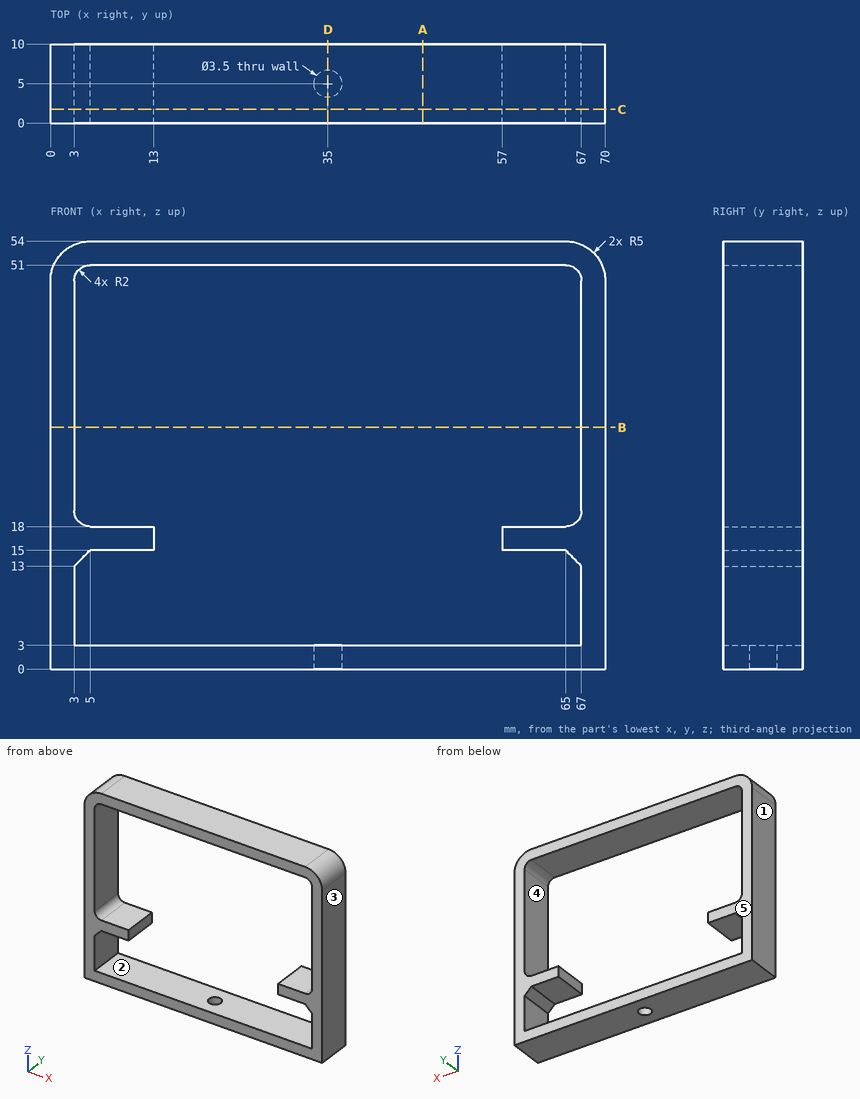
Study the drawing (mm; zero at the part's minimum x, y, z) and answer. A direction names the side the tool comes from. Round coordinates to 2 decimals unless told otherwise and drop trailing zeros. Write each loop counter-clockwise with the first axis right and the second up, starting at its lowest first coordinate (ties: lowest second). Pieces come first, ordered by that corner, then holes. Notation, with made-up numbers: (53.5, -23.75) -> (98.5, -23.75) arc R17 cw to (98.5, 5.25) -> close; hole circle Ø10 at (-4.75, -5). An arc over 180 degrees is marked (long way). Write item = value, one per line.
1) Which of the six approach directions +Z, -Z, +X, -X, +Y, -Y give full straight-line access (tool end or side, diameter ignored) to the marked faces 4 and 5?
Check values:
face_4 = +Y, -Y
face_5 = +Z, -Z, +X, -X, +Y
2) For a pull along X with two mould halves and no side action, classify the marked faces 1, 2 and 3 as released by +X, released by -X, zero draft, split by the parting line, or undercut.
Check values:
face_1 = released by -X
face_2 = undercut
face_3 = released by +X
3) Given pin 1 (2.5 mm diameter, centred on x = 61, y = 6, fed in from -Z); pin 2 (8 mm diameter, centred on x = 8.5, z = 32, fed in from +Y), each flat-ended and moving along its own axis, determine where each tip first touches the part or whether it passes through.
Check values:
pin_1 = 0
pin_2 = through
4) Section B-B on z = 30.5 is taken. Write down the section's boundary in (x, y).
Check values:
outline = (0, 0) -> (3, 0) -> (3, 10) -> (0, 10) -> close; (67, 0) -> (70, 0) -> (70, 10) -> (67, 10) -> close
5) Straight lines are drawn through the part: line 1 along Z through (x, y) = (60, 5); line 2 along Z through (x, y) = (48, 8); line 3 along Y through (x, z) = (35, 1.1). For each, find the intervals that lie inside material, in ascending order. Write a range as [from, to].
Check values:
line_1 = [0, 3], [15, 18], [51, 54]
line_2 = [0, 3], [51, 54]
line_3 = [0, 3.25], [6.75, 10]
6) Section A-A on x = 47 is taken. Write down the section's boundary in (y, z).
Check values:
outline = (0, 0) -> (10, 0) -> (10, 3) -> (0, 3) -> close; (0, 51) -> (10, 51) -> (10, 54) -> (0, 54) -> close
7) Section D-D on x = 35 is taken. Write down the section's boundary in (y, z).
Check values:
outline = (0, 0) -> (3.25, 0) -> (3.25, 3) -> (0, 3) -> close; (0, 51) -> (10, 51) -> (10, 54) -> (0, 54) -> close; (6.75, 0) -> (10, 0) -> (10, 3) -> (6.75, 3) -> close
8) Section C-C on y = 1.75 is taken. Write down the section's boundary in (x, z), plus the area to 3 significant figures.
Check values:
outline = (0, 0) -> (70, 0) -> (70, 49) arc R5 ccw to (65, 54) -> (5, 54) arc R5 ccw to (0, 49) -> close; hole (3, 3) -> (67, 3) -> (67, 13) -> (65, 15) -> (57, 15) -> (57, 18) -> (65, 18) arc R2 ccw to (67, 20) -> (67, 49) arc R2 ccw to (65, 51) -> (5, 51) arc R2 ccw to (3, 49) -> (3, 20) arc R2 ccw to (5, 18) -> (13, 18) -> (13, 15) -> (5, 15) -> (3, 13) -> close
area = 765 mm²
